Source: CAD feature listing. Evaluate the final solid. Frame: model axes, mm. Face numbers are marked on the shaded views. Round coordinates to 2 decimals unless told otherwise and drop trailing zeros. Write each loop counter-clockwise with the first axis right and the second up, starting at its lowest first coordinate (ties: lowest second). Pieces come first, ordered by that corner, then holes.
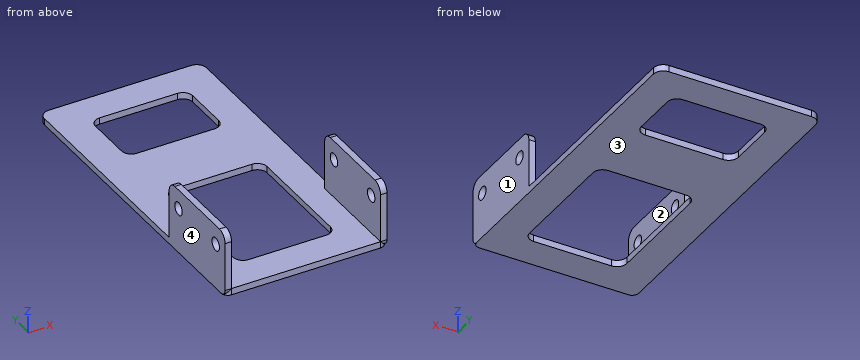
from build123d import *

# Parameters (mm, degrees)
CYLINDER003_R     = 2
CYLINDER003_DEPTH = 10
CYLINDER002_R     = 2
CYLINDER002_DEPTH = 10
BOX007_W          = 2
BOX007_H          = 30
BOX007_DEPTH      = 20
FILLET009_R       = 2
FILLET010_R       = 3
BOX006_W          = 30
BOX006_H          = 20
BOX006_DEPTH      = 2
FILLET008_R       = 3
BOX005_W          = 30
BOX005_H          = 40
BOX005_DEPTH      = 2
FILLET007_R       = 3
BOX004_W          = 50
BOX004_H          = 100
BOX004_DEPTH      = 2
FILLET005_R       = 2
FILLET006_R       = 3
CYLINDER005_R     = 2
CYLINDER005_DEPTH = 10
CYLINDER004_R     = 2
CYLINDER004_DEPTH = 10
BOX008_W          = 2
BOX008_H          = 30
BOX008_DEPTH      = 20
FILLET011_R       = 2
FILLET012_R       = 3


with BuildPart() as cylinder003:
    # Cylinder003 → Cylinder003 (new body)
    with BuildSketch(Plane(origin=(0, 25, 14), x_dir=(0, 0, -1), z_dir=(1, 0, 0))):
        Circle(CYLINDER003_R)
    extrude(amount=CYLINDER003_DEPTH)


with BuildPart() as cylinder002:
    # Cylinder002 → Cylinder002 (new body)
    with BuildSketch(Plane(origin=(0, 5, 14), x_dir=(0, 0, -1), z_dir=(1, 0, 0))):
        Circle(CYLINDER002_R)
    extrude(amount=CYLINDER002_DEPTH)


with BuildPart() as mini_pe_a:
    # Box007 → Box007 (new body)
    with BuildSketch(Plane.XY):
        with Locations((1, 15)):
            Rectangle(BOX007_W, BOX007_H)
    extrude(amount=BOX007_DEPTH)

    # Fillet009
    fillet009_edges = [mini_pe_a.edges().sort_by_distance(p)[0] for p in [
        (1, 0, 0),
        (1, 30, 0),
    ]]
    fillet(fillet009_edges, radius=FILLET009_R)

    # Fillet010
    fillet010_edges = [mini_pe_a.edges().sort_by_distance(p)[0] for p in [
        (1, 0, 20),
        (1, 30, 20),
    ]]
    fillet(fillet010_edges, radius=FILLET010_R)

    # Cut006: cut Cylinder002
    add(cylinder002.part, mode=Mode.SUBTRACT)

    # Cut007: cut Cylinder003
    add(cylinder003.part, mode=Mode.SUBTRACT)


with BuildPart() as forat2:
    # Box006 → Box006 (new body)
    with BuildSketch(Plane.XY):
        with Locations((15, 10)):
            Rectangle(BOX006_W, BOX006_H)
    extrude(amount=BOX006_DEPTH)

    # Fillet008
    fillet008_edges = [forat2.edges().sort_by_distance(p)[0] for p in [
        (0, 0, 1),
        (0, 20, 1),
        (30, 0, 1),
        (30, 20, 1),
    ]]
    fillet(fillet008_edges, radius=FILLET008_R)


with BuildPart() as forat2_1:
    # Fillet008 placement: moved
    add(forat2.part.moved(Location((10, 70, 0))))


with BuildPart() as forat1:
    # Box005 → Box005 (new body)
    with BuildSketch(Plane.XY):
        with Locations((15, 20)):
            Rectangle(BOX005_W, BOX005_H)
    extrude(amount=BOX005_DEPTH)

    # Fillet007
    fillet007_edges = [forat1.edges().sort_by_distance(p)[0] for p in [
        (0, 0, 1),
        (0, 40, 1),
        (30, 0, 1),
        (30, 40, 1),
    ]]
    fillet(fillet007_edges, radius=FILLET007_R)


with BuildPart() as forat1_1:
    # Fillet007 placement: moved
    add(forat1.part.moved(Location((10, 10, 0))))


with BuildPart() as fusion:
    # Box004 → Box004 (new body)
    with BuildSketch(Plane.XY):
        with Locations((25, 50)):
            Rectangle(BOX004_W, BOX004_H)
    extrude(amount=BOX004_DEPTH)

    # Fillet005
    fillet005_edges = [fusion.edges().sort_by_distance(p)[0] for p in [
        (0, 0, 1),
        (50, 0, 1),
    ]]
    fillet(fillet005_edges, radius=FILLET005_R)

    # Fillet006
    fillet006_edges = [fusion.edges().sort_by_distance(p)[0] for p in [
        (0, 100, 1),
        (50, 100, 1),
    ]]
    fillet(fillet006_edges, radius=FILLET006_R)

    # Cut004: cut forat1
    add(forat1_1.part, mode=Mode.SUBTRACT)

    # Cut005: cut forat2
    add(forat2_1.part, mode=Mode.SUBTRACT)

    add(mini_pe_a.part)


with BuildPart() as cylinder005:
    # Cylinder005 → Cylinder005 (new body)
    with BuildSketch(Plane(origin=(0, 25, 14), x_dir=(0, 0, -1), z_dir=(1, 0, 0))):
        Circle(CYLINDER005_R)
    extrude(amount=CYLINDER005_DEPTH)


with BuildPart() as cylinder004:
    # Cylinder004 → Cylinder004 (new body)
    with BuildSketch(Plane(origin=(0, 5, 14), x_dir=(0, 0, -1), z_dir=(1, 0, 0))):
        Circle(CYLINDER004_R)
    extrude(amount=CYLINDER004_DEPTH)


with BuildPart() as pe_a:
    # Box008 → Box008 (new body)
    with BuildSketch(Plane.XY):
        with Locations((1, 15)):
            Rectangle(BOX008_W, BOX008_H)
    extrude(amount=BOX008_DEPTH)

    # Fillet011
    fillet011_edges = [pe_a.edges().sort_by_distance(p)[0] for p in [
        (1, 0, 0),
        (1, 30, 0),
    ]]
    fillet(fillet011_edges, radius=FILLET011_R)

    # Fillet012
    fillet012_edges = [pe_a.edges().sort_by_distance(p)[0] for p in [
        (1, 0, 20),
        (1, 30, 20),
    ]]
    fillet(fillet012_edges, radius=FILLET012_R)

    # Cut008: cut Cylinder004
    add(cylinder004.part, mode=Mode.SUBTRACT)

    # Cut009: cut Cylinder005
    add(cylinder005.part, mode=Mode.SUBTRACT)


with BuildPart() as pe_a_1:
    # Cut009 placement: moved
    add(pe_a.part.moved(Location((48, 0, 0))))

    # Fusion001: union Fusion
    add(fusion.part)


solid = pe_a_1.part
1) Section query A-A on y = 18.5. Return the cut outline in (x, z).
Taken from the geometry:
outline: (0, 0) - (10, 0) - (10, 2) - (2, 2) - (2, 20) - (0, 20) - close; (40, 0) - (50, 0) - (50, 20) - (48, 20) - (48, 2) - (40, 2) - close
2) Section query C-C on y = 5. Return the cut outline in (x, z).
Taken from the geometry:
outline: (0, 0) - (50, 0) - (50, 12) - (48, 12) - (48, 2) - (2, 2) - (2, 12) - (0, 12) - close; (0, 16) - (2, 16) - (2, 20) - (0, 20) - close; (48, 16) - (50, 16) - (50, 20) - (48, 20) - close
3) Section query B-B on x = 32. Return the cut outline in (y, z), then the cut area to 3 significant figures.
Taken from the geometry:
outline: (0, 0) - (10, 0) - (10, 2) - (0, 2) - close; (50, 0) - (70, 0) - (70, 2) - (50, 2) - close; (90, 0) - (100, 0) - (100, 2) - (90, 2) - close
area: 80.0 mm2
4) Contact query for flat-ended pins moving along their axis: P1, Ø25, axis at x = 25, y = 46, coming from the +Z side; P2, Ø0.6, axis at x = 49, z = 11.5, coming from the +Y side. Output: stop coordinate, or through.
Taken from the geometry:
P1: stops at z = 2
P2: stops at y = 30
5) Material intervals for line 1 (Y direction, x = 48.8, z = 14); line 2 (Z direction, x = 1.25, y = 5); line 3 (X direction, y = 29, z = 12.5), sorted ascending.
Taken from the geometry:
line 1: y = 0 to 3, 7 to 23, 27 to 30
line 2: z = 0 to 12, 16 to 20
line 3: x = 0 to 2, 48 to 50
6) Section query D-D on z = 14. Return the cut outline in (x, y), then the cut area to 3 significant figures.
Taken from the geometry:
outline: (0, 0) - (2, 0) - (2, 3) - (0, 3) - close; (0, 7) - (2, 7) - (2, 23) - (0, 23) - close; (0, 27) - (2, 27) - (2, 30) - (0, 30) - close; (48, 0) - (50, 0) - (50, 3) - (48, 3) - close; (48, 7) - (50, 7) - (50, 23) - (48, 23) - close; (48, 27) - (50, 27) - (50, 30) - (48, 30) - close
area: 88.0 mm2
7) Pull-direction query (X, two-part tool) for the marked faces 1, 2, 3 and 4; classes: released by +X, released by -X, zero draft, split by the parting line, or undercut.
Taken from the geometry:
face 1: released by +X
face 2: undercut
face 3: zero draft
face 4: released by -X
